Geometry: final body of the model. Coordinates: model frame, mm. A direction names the side the tool comes from. Give positions to 0.01 mm unless a question says otherwise; leave off trailing zeros. Loops run counter-clockwise (first coordinate to the right, second up) from the corner with the lowest first, then second, coordinate; pieces in that order, holes last.
from build123d import *

# Parameters (mm, degrees)
F0_R     = 11.9904594856
F0_R_2   = 3
F1_DEPTH = 3


with BuildPart() as f1:
    # F0 (on Top) → F1 (new body)
    with BuildSketch(Plane.XY):
        with BuildLine():
            ThreePointArc((-12.1153572012, -14.7200148072), (-3.4183411814, -9.5323228549), (0, 0))
            ThreePointArc((0, 0), (-3.8709155487, 10.0570114485), (-13.4857972368, 14.9233772985))
            ThreePointArc((-13.4857972368, 14.9233772985), (-29.9808320776, 0.7580700902), (-15, -15))
            Line((-15, -15), (-12.1153572012, -14.7200148072))
        make_face()
        with Locations((-15, 0)):
            Circle(F0_R, mode=Mode.SUBTRACT)
        with BuildLine():
            ThreePointArc((-13.4857972368, 14.9233772985), (-3.8709155487, 10.0570114485), (0, 0))
            ThreePointArc((0, 0), (-3.4183411814, -9.5323228549), (-12.1153572012, -14.7200148072))
            Line((-12.1153572012, -14.7200148072), (36.5142027632, -10))
            ThreePointArc((36.5142027632, -10), (26.5142027632, 0), (36.5142027632, 10))
            Line((36.5142027632, 10), (-13.4857972368, 14.9233772985))
        make_face()
        with Locations((6.2150359154, 0)):
            Circle(F0_R_2, mode=Mode.SUBTRACT)
        with Locations((14.6543458104, 0)):
            Circle(F0_R_2, mode=Mode.SUBTRACT)
        with Locations((22.0015123487, 0)):
            Circle(F0_R_2, mode=Mode.SUBTRACT)
        with BuildLine():
            ThreePointArc((-15, -15), (-13.5509006431, -14.9298396192), (-12.1153572012, -14.7200148072))
            Line((-12.1153572012, -14.7200148072), (-15, -15))
        make_face()
        with BuildLine():
            ThreePointArc((44.0375149849, 6.5878504245), (40.6446685817, 9.107098996), (36.5142027632, 10))
            ThreePointArc((36.5142027632, 10), (26.5142027632, 0), (36.5142027632, -10))
            ThreePointArc((36.5142027632, -10), (39.7671043031, -9.4561425313), (42.6661828836, -7.8837263143))
            Line((42.6661828836, -7.8837263143), (43.5123325587, -7.1432611156))
            ThreePointArc((43.5123325587, -7.1432611156), (45.7332400761, -3.8741903699), (46.5142027632, 0))
            ThreePointArc((46.5142027632, 0), (45.8745746099, 3.5190110673), (44.0375149849, 6.5878504245))
        make_face()
        with BuildLine():
            ThreePointArc((43.3583631677, 0), (30.1078141267, -2.408467621), (41.6632783251, 4.5088305026))
            ThreePointArc((41.6632783251, 4.5088305026), (42.9205913997, 2.408467621), (43.3583631677, 0))
        make_face(mode=Mode.SUBTRACT)
        with BuildLine():
            Line((66.2282739463, 39.0671108823), (36.5142027632, 10))
            ThreePointArc((36.5142027632, 10), (40.6446685817, 9.107098996), (44.0375149849, 6.5878504245))
            Line((44.0375149849, 6.5878504245), (44.8677292107, 7.3148343617))
            ThreePointArc((44.8677292107, 7.3148343617), (45.1483677498, 11.5481831556), (49.3817165437, 11.2675446164))
            Line((49.3817165437, 11.2675446164), (53.0654896509, 14.4932709338))
            ThreePointArc((53.0654896509, 14.4932709338), (53.34612819, 18.7266197277), (57.5794769839, 18.4459811885))
            Line((57.5794769839, 18.4459811885), (60.8896796087, 21.3445874307))
            ThreePointArc((60.8896796087, 21.3445874307), (61.1703181479, 25.5779362245), (65.4036669417, 25.2972976854))
            Line((65.4036669417, 25.2972976854), (66.6074516499, 26.3514016979))
            ThreePointArc((66.6074516499, 26.3514016979), (64.7703920248, 29.4202410551), (64.1307638715, 32.9392521224))
            ThreePointArc((64.1307638715, 32.9392521224), (64.669661947, 36.1777008828), (66.2282739463, 39.0671108823))
        make_face()
        with BuildLine():
            Line((44.8677292107, 7.3148343617), (44.0375149849, 6.5878504245))
            ThreePointArc((44.0375149849, 6.5878504245), (45.8745746099, 3.5190110673), (46.5142027632, 0))
            ThreePointArc((46.5142027632, 0), (45.7332400761, -3.8741903699), (43.5123325587, -7.1432611156))
            Line((43.5123325587, -7.1432611156), (80.7162342327, 25.4138564436))
            ThreePointArc((80.7162342327, 25.4138564436), (73.4677143901, 22.9612580662), (66.6074516499, 26.3514016979))
            Line((66.6074516499, 26.3514016979), (65.4036669417, 25.2972976854))
            ThreePointArc((65.4036669417, 25.2972976854), (65.9547848292, 24.3766458782), (66.1466732752, 23.320942558))
            ThreePointArc((66.1466732752, 23.320942558), (64.2023765954, 20.512831004), (60.8896796087, 21.3445874307))
            Line((60.8896796087, 21.3445874307), (57.5794769839, 18.4459811885))
            ThreePointArc((57.5794769839, 18.4459811885), (58.1305948714, 17.5253293814), (58.3224833174, 16.4696260612))
            ThreePointArc((58.3224833174, 16.4696260612), (56.3781866375, 13.6615145072), (53.0654896509, 14.4932709338))
            Line((53.0654896509, 14.4932709338), (49.3817165437, 11.2675446164))
            ThreePointArc((49.3817165437, 11.2675446164), (49.9328344312, 10.3468928092), (50.1247228772, 9.2911894891))
            ThreePointArc((50.1247228772, 9.2911894891), (48.1804261974, 6.4830779351), (44.8677292107, 7.3148343617))
        make_face()
        with BuildLine():
            Line((66.1307166189, 38.7820979372), (66.2282739463, 39.0671108823))
            ThreePointArc((66.2282739463, 39.0671108823), (64.669661947, 36.1777008828), (64.1307638715, 32.9392521224))
            Line((64.1307638715, 32.9392521224), (64.228321199, 33.2242650675))
            ThreePointArc((64.228321199, 33.2242650675), (64.7580821351, 36.1474354602), (66.1307166189, 38.7820979372))
        make_face()
        with BuildLine():
            ThreePointArc((84.1307638715, 32.9392521224), (77.369212632, 42.4003540469), (66.2282739463, 39.0671108823))
            Line((66.2282739463, 39.0671108823), (66.1307166189, 38.7820979372))
            ThreePointArc((66.1307166189, 38.7820979372), (77.2037744065, 42.3571186277), (84.0373073283, 32.9392521224))
            ThreePointArc((84.0373073283, 32.9392521224), (77.6168874778, 23.6663590753), (66.6777619252, 26.4129694707))
            Line((66.6777619252, 26.4129694707), (66.6074516499, 26.3514016979))
            ThreePointArc((66.6074516499, 26.3514016979), (73.4677143901, 22.9612580662), (80.7162342327, 25.4138564436))
            ThreePointArc((80.7162342327, 25.4138564436), (83.2372094902, 28.8073460012), (84.1307638715, 32.9392521224))
        make_face()
        with BuildLine():
            Line((43.5123325587, -7.1432611156), (42.6661828836, -7.8837263143))
            ThreePointArc((42.6661828836, -7.8837263143), (43.0996731243, -7.5253956788), (43.5123325587, -7.1432611156))
        make_face()
    extrude(amount=F1_DEPTH)


solid = f1.part
Item 1: Section query A-A on x = -17. Return loops of the section in (y, z).
Values follow:
outline: (-14.87, 0) - (-11.82, 0) - (-11.82, 3) - (-14.87, 3) - close; (11.82, 0) - (14.87, 0) - (14.87, 3) - (11.82, 3) - close
Item 2: Section query B-B on z = 1.95. Give the number of separate pieces and of enclosed holes in the cut face, plus the area to 3 significant figures.
Values follow:
separate pieces: 1
enclosed holes: 9
area: 1,660 mm2
Item 3: Ray query, probe 1 along X at (y, z) = (4.5, 2.65); probe 2 along Y at (x, z) = (65, 0.1); probe 3 along X at (y, z) = (5.5, 0.4). Return the intervals inside material, ascending.
Values follow:
probe 1: x = -29.31 to -26.11, -3.89 to 31.36, 41.67 to 56.82
probe 2: y = 11.66 to 20.96, 25.68 to 28.86, 36.78 to 37.87
probe 3: x = -28.96 to -25.65, -4.35 to 32.44, 40.59 to 57.96
Item 4: Section query C-C on x = 23. Return loops of the section in (y, z), plus the area to 3 significant figures.
Values follow:
outline: (-11.31, 0) - (-2.83, 0) - (-2.83, 3) - (-11.31, 3) - close; (2.83, 0) - (11.33, 0) - (11.33, 3) - (2.83, 3) - close
area: 51.0 mm2
Item 5: Pin query (flat end, axial travel): pin 1 (8 mm diameter, centred on x = 36.51, y = 0, fed in from +Z); pin 2 (1.5 mm diameter, centred on x = 63, z = 0.5, fed in from -Y); pin 3 (1.5 mm diameter, centred on x = 22, z = 2, fed in from -Y); pin 4 (1.5 mm diameter, centred on x = 9, y = 3, fed in from -Z). Return the tip coordinate at first contact, or that it passes through.
Values follow:
pin 1: passes through
pin 2: stops at y = 9.25
pin 3: stops at y = -11.48
pin 4: stops at z = 0
Item 6: Set-up query: faces 4 (the face through (11.864, 12.427, 1.479)), 5 (the face through (23, 6, 0)), 6 (the face through (64.79, 29.37, 1.48)). Return all of +Z, -Z, +X, -X, +Y, -Y with unobstructed straight access to the full face (end or side cutting, diameter ignored); none if empty.
Values follow:
face 4: +Z, -Z, +Y
face 5: -Z, +X, -X, +Y, -Y
face 6: +Z, -Z
Item 7: Draft query along Y for faces 1 (the face through (-3.563, 3.602, 1.479)), 2 (the face through (51.58, 24.74, 1.48)), 3 (the face through (61.854, 8.907, 1.479)). Return one class per face: +Y half, -Y half, draft (parallel to the pull), parting line (faces both ways), or undercut.
Values follow:
face 1: undercut
face 2: +Y half
face 3: -Y half
